Here's how the part is built. I have some questions about the finished solid (model axes, mm). Round coordinates to 2 decimals unless told otherwise and drop trailing zeros. Write each loop counter-clockwise with the first axis right and the second up, starting at its lowest first coordinate (ties: lowest second). Pieces come first, ordered by that corner, then holes. Notation, with made-up numbers: (17.5, -30) - (29.5, -30) arc R11 ccw to (29.5, -15) - close; hole circle Ø1 at (32.25, -10.5). An arc over 180 degrees is marked (long way). Return JSON: item names as keys, results as strings. Group by question number.
```python
from build123d import *

# Parameters (mm, degrees)
SKETCH1_W           = 400
SKETCH1_H           = 200
SKETCH1_R           = 4.75
SKETCH1_R_2         = 57.5
BOSS_EXTRUDE1_DEPTH = 10
SKETCH2_R           = 3.1
CUT_EXTRUDE1_DEPTH  = 10


with BuildPart() as part:
    # Sketch1 → Boss-Extrude1 (new body)
    with BuildSketch(Plane.XY):
        Rectangle(SKETCH1_W, SKETCH1_H)
        with Locations((-52.757236944, 52.757236944)):
            Circle(SKETCH1_R, mode=Mode.SUBTRACT)
        with Locations((52.757236944, 52.757236944)):
            Circle(SKETCH1_R, mode=Mode.SUBTRACT)
        with Locations((52.757236944, -52.757236944)):
            Circle(SKETCH1_R, mode=Mode.SUBTRACT)
        with Locations((-52.757236944, -52.757236944)):
            Circle(SKETCH1_R, mode=Mode.SUBTRACT)
        Circle(SKETCH1_R_2, mode=Mode.SUBTRACT)
    extrude(amount=BOSS_EXTRUDE1_DEPTH)

    # Sketch2 → Cut-Extrude1 (cut)
    with BuildSketch(Plane.XY.offset(10)):
        with Locations((-185, 85)):
            Circle(SKETCH2_R)
        with Locations((-185, 28.333333333)):
            Circle(SKETCH2_R)
        with Locations((-185, -85)):
            Circle(SKETCH2_R)
        with Locations((-185, -28.333333333)):
            Circle(SKETCH2_R)
        with Locations(Location((185, -28.333333333, 0), (0, 0, 180))):
            Circle(SKETCH2_R)
        with Locations(Location((185, -85, 0), (0, 0, 180))):
            Circle(SKETCH2_R)
        with Locations(Location((185, 28.333333333, 0), (0, 0, 180))):
            Circle(SKETCH2_R)
        with Locations(Location((185, 85, 0), (0, 0, 180))):
            Circle(SKETCH2_R)
        with Locations((-111, 85)):
            Circle(SKETCH2_R)
        with Locations((-37, 85)):
            Circle(SKETCH2_R)
        with Locations((37, 85)):
            Circle(SKETCH2_R)
        with Locations((111, 85)):
            Circle(SKETCH2_R)
    extrude(amount=-CUT_EXTRUDE1_DEPTH, mode=Mode.SUBTRACT)


solid = part.part
```
1) Imagine slicing it at B-B (x = 0). Please give me the cut outline in (y, z), plus the area to 3 significant figures.
2) Imagine slicing it at A-A (y = 0). Please give me the cut outline in (x, z), plus the area to 3 significant figures.
3) If we mould it in two halves opening along Y, with no side actions, what happens to faces 1 (the cylindrical face through (-50.57, 48.54, 4.93)), 2 (the flat face through (-47, 46, 0)), 3 (the flat face through (-3, 100, 5))? For each: released by +Y, released by -Y, zero draft, split by the parting line, or undercut.
4) Will these pins go through, and if not, where does the flat tip stop? pin 1 Ø3.5 at (x, y) = (185, 28.33) entering from -Z; pin 2 Ø7 at (x, y) = (37, 85) entering from -Z.
5) Imagine slicing it at C-C (z = 8.5). Give the number of separate pieces and of enclosed holes in the cut face, plus the area to 3 significant figures.
6) I need wall thicknesses on line 1 along Y through (x, z) = (185, 2.25); line 2 along Y through (x, z) = (-0.5, 2.75); line 3 along X through (y, z) = (49, 9.75). Which ranges of each line are inside material? Lowest first, please.
Results found:
{
 "1": {"outline": "(-100, 0) - (-57.5, 0) - (-57.5, 10) - (-100, 10) - close; (57.5, 0) - (100, 0) - (100, 10) - (57.5, 10) - close", "area": "850 mm²"},
 "2": {"outline": "(-200, 0) - (-57.5, 0) - (-57.5, 10) - (-200, 10) - close; (57.5, 0) - (200, 0) - (200, 10) - (57.5, 10) - close", "area": "2,850 mm²"},
 "3": {"face 1": "undercut", "face 2": "zero draft", "face 3": "released by +Y"},
 "4": {"pin 1": "passes through", "pin 2": "stops at z = 0"},
 "5": {"separate pieces": "1", "enclosed holes": "17", "area": "69,000 mm²"},
 "6": {"line 1": "y = -100 to -88.1, -81.9 to -31.43, -25.23 to 25.23, 31.43 to 81.9, 88.1 to 100", "line 2": "y = -100 to -57.5, 57.5 to 100", "line 3": "x = -200 to -55.66, -49.85 to -30.09, 30.09 to 49.85, 55.66 to 200"}
}
